Geometry check sheet. Reference: the model listing, model coordinates, mm. Round coordinates to 2 decimals unless told otherwise and drop trailing zeros. Order: outer loops, then holes, each group sorted by start corner. A loop starts at its lowest first (then second) coordinate and runs counter-clockwise, first axis right, second up.
```python
from build123d import *

# Parameters (mm, degrees)
F1_DEPTH = 0.5
F3_DEPTH = 0.501
F5_DEPTH = 0.501


with BuildPart() as f1:
    # F0 (on Top) → F1 (new body)
    with BuildSketch(Plane.XY):
        Polygon((6.25, -10.825318), (12.5, 0), (6.25, 10.825318), (-6.25, 10.825318), (-12.5, 0), (-6.25, -10.825318), align=None)
    extrude(amount=F1_DEPTH)

    # F2 (on face) → F3 (cut, through all)
    with BuildSketch(Plane.XY.offset(0.5)):
        with BuildLine():
            ThreePointArc((3.216667, -10.825318), (3.040931, -10.401053), (2.616667, -10.225318))
            Line((2.616667, -10.225318), (2.116667, -10.225318))
            ThreePointArc((2.116667, -10.225318), (1.692403, -10.401053), (1.516667, -10.825318))
            Line((1.516667, -10.825318), (3.216667, -10.825318))
        make_face()
        with BuildLine():
            Line((-3.216667, -10.825318), (-1.516667, -10.825318))
            ThreePointArc((-1.516667, -10.825318), (-1.692403, -10.401053), (-2.116667, -10.225318))
            Line((-2.116667, -10.225318), (-2.616667, -10.225318))
            ThreePointArc((-2.616667, -10.225318), (-3.040931, -10.401053), (-3.216667, -10.825318))
        make_face()
    extrude(amount=-F3_DEPTH, mode=Mode.SUBTRACT)

    # F4 (on face) → F5 (cut, through all)
    with BuildSketch(Plane.XY.offset(0.5)):
        Polygon((-6.25, 10.825318), (-12.5, 0), (12.5, 0), (6.25, 10.825318), align=None)
    extrude(amount=-F5_DEPTH, mode=Mode.SUBTRACT)


solid = f1.part
```
(1) Sectioned sample at C-C, the plane y = -5.5. Record the cut outline in (x, z), and give its area (3 significant figures).
Returned:
outline: (-9.32, 0) - (9.32, 0) - (9.32, 0.5) - (-9.32, 0.5) - close
area: 9.32 mm2
(2) Sectioned sample at B-B, the plane x = 9.25. Record the cut outline in (y, z).
Returned:
outline: (-5.63, 0) - (0, 0) - (0, 0.5) - (-5.63, 0.5) - close
(3) Material ranges on line 1 (X direction, y = -8, z = 0.4); line 2 (X direction, y = -2, z = 0.1); line 3 (Y direction, x = -8.25, z = 0.2), recorded low to high.
Returned:
line 1: x = -7.88 to 7.88
line 2: x = -11.35 to 11.35
line 3: y = -7.36 to 0
(4) Draft check along X on faces 1 (the flat face through (-9.419, -5.337, 0.246)), 2 (the flat face through (0, -4, 0)), 3 (the flat face through (9.33, -5.49, 0.25)). Enter one of: released by +X, released by -X, zero draft, split by the parting line, or undercut.
Returned:
face 1: released by -X
face 2: zero draft
face 3: released by +X
(5) Sectioned sample at A-A, the plane z = 0.15. Record the cut outline in (x, y), and give its area (3 significant figures).
Returned:
outline: (-12.5, 0) - (-6.25, -10.83) - (-3.22, -10.83) arc R0.6 cw to (-2.62, -10.23) - (-2.12, -10.23) arc R0.6 cw to (-1.52, -10.83) - (1.52, -10.83) arc R0.6 cw to (2.12, -10.23) - (2.62, -10.23) arc R0.6 cw to (3.22, -10.83) - (6.25, -10.83) - (12.5, 0) - close
area: 201 mm2
